Geometry: final body of the model. Coordinates: model frame, mm. A direction names the side the tool comes from. Give positions to 0.01 mm unless a question says otherwise; leave off trailing zeros. Loops run counter-clockwise (first coordinate to the right, second up) from the corner with the lowest first, then second, coordinate; pieces in that order, holes last. Notation, with made-up numbers: (-8.5, -4) -> (37.5, -4) arc R21 ccw to (37.5, 17) -> close; hole circle Ø3 at (68, 77). An arc over 180 degrees is marked (long way). Answer in a Markdown table with one row per item. Add a question column.
1) Section query D-D (x = 7.75). Return the cut outline in (y, z).
2) First-contact query: P1, Ø4, axis at y = 1, z = 6.5, coming from the +X side; P2, Ø3.5, axis at x = 2.5, z = 5.5, coming from the +Y side. Flat tips, straight axial feed; report the tip coordinate or a pass-through.
3) Section query A-A (x = 4.25). Return the cut outline in (y, z).
4) Line query: line 1 (X direction, y = 1.25, z = 6.5); line 2 (Z direction, x = 3.5, y = -2); line 3 (Y direction, x = -6.5, z = 7.75). Output: solid intervals per line, ascending. Write a range as from..to.
5) Section query C-C (y = 1.25). Return the cut outline in (x, z), plus the area to 3 significant figures.
6) Draft query along Z for faces 5 (the flat face through (0, 0, 2)), 6 (the cylindrical face through (6.715, -0.035, 8.699)), 7 (the flat face through (0, 10, 1)). Return one class per face: +Z half, -Z half, draft (parallel to the pull), parting line (faces both ways), or undercut.
7) Access query for faces 1 (the flat face through (-7, 0, 6)), 2 (the flat face through (5, 0, 5)), 3 (the flat face through (7, 0, 5)), 4 (the flat face through (2, -2.5, 8)). Directions: +Z, -Z, +X, -X, +Y, -Y. A direction counts if a zero-diameter tool reaches every point of the face in a straight line with its end or side. Return the directions, or none.
8) Section query B-B (z = 2.75). Return the cut outline in (x, y), plus the area to 3 significant figures.
```python
from build123d import *

# Parameters (mm, degrees)
SKETCH_W        = 20
SKETCH_H        = 20
PAD_DEPTH       = 2
PAD001_DEPTH    = 2.5
CHAMFER_SIZE    = 1
CHAMFER001_SIZE = 1
FILLET_R        = 1
FILLET001_R     = 1
FILLET002_R     = 1


with BuildPart() as part:
    # Sketch → Pad (new body)
    with BuildSketch(Plane.XY):
        Rectangle(SKETCH_W, SKETCH_H)
    extrude(amount=PAD_DEPTH)

    # Sketch001 → Pad001 (join, symmetric)
    with BuildSketch(Plane.XZ):
        Polygon((-5, 2), (-5, 7), (5, 7), (5, 1.996067), (7, 1.996067), (7, 9), (-7, 9), (-7, 2), align=None)
    extrude(amount=PAD001_DEPTH, both=True)

    # Chamfer
    chamfer_edges = [part.edges().sort_by_distance(p)[0] for p in [
        (7, 0, 2),
    ]]
    chamfer(chamfer_edges, length=CHAMFER_SIZE)

    # Chamfer001
    chamfer001_edges = [part.edges().sort_by_distance(p)[0] for p in [
        (-7, 0, 2),
    ]]
    chamfer(chamfer001_edges, length=CHAMFER001_SIZE)

    # Fillet
    fillet_edges = [part.edges().sort_by_distance(p)[0] for p in [
        (-10, 10, 1),
    ]]
    fillet(fillet_edges, radius=FILLET_R)

    # Fillet001
    fillet001_edges = [part.edges().sort_by_distance(p)[0] for p in [
        (10, -10, 1),
        (-10, -10, 1),
        (10, 10, 1),
    ]]
    fillet(fillet001_edges, radius=FILLET001_R)

    # Fillet002
    fillet002_edges = [part.edges().sort_by_distance(p)[0] for p in [
        (7, 0, 9),
        (-7, 0, 9),
    ]]
    fillet(fillet002_edges, radius=FILLET002_R)


solid = part.part
```
Evaluation:
| question | item | result |
|---|---|---|
| 1 | outline | (-10, 0) -> (10, 0) -> (10, 2) -> (2.5, 2) -> (2.5, 2.25) -> (-2.5, 2.25) -> (-2.5, 2) -> (-10, 2) -> close |
| 2 | P1 | x = 7 |
| 2 | P2 | y = 2.5 |
| 3 | outline | (-10, 0) -> (10, 0) -> (10, 2) -> (-10, 2) -> close; (-2.5, 7) -> (2.5, 7) -> (2.5, 9) -> (-2.5, 9) -> close |
| 4 | line 1 | -7..-5, 5..7 |
| 4 | line 2 | 0..2, 7..9 |
| 4 | line 3 | -2.5..2.5 |
| 5 | outline | (-10, 0) -> (10, 0) -> (10, 2) -> (8, 2) -> (7, 3) -> (7, 8) arc R1 ccw to (6, 9) -> (-6, 9) arc R1 ccw to (-7, 8) -> (-7, 3) -> (-8, 2) -> (-10, 2) -> close; hole (-5, 2) -> (5, 2) -> (5, 7) -> (-5, 7) -> close |
| 5 | area | 88.6 mm² |
| 6 | face 5 | undercut |
| 6 | face 6 | +Z half |
| 6 | face 7 | draft |
| 7 | face 1 | +Z, -X, +Y, -Y |
| 7 | face 2 | +Y, -Y |
| 7 | face 3 | +Z, +X, +Y, -Y |
| 7 | face 4 | +Z, +X, -X, -Y |
| 8 | outline | (-7.25, -2.5) -> (-5, -2.5) -> (-5, 2.5) -> (-7.25, 2.5) -> close; (5, -2.5) -> (7.25, -2.5) -> (7.25, 2.5) -> (5, 2.5) -> close |
| 8 | area | 22.5 mm² |
